```python
from build123d import *

# Parameters (mm, degrees)
SKETCH1_W           = 200
SKETCH1_H           = 120
BOSS_EXTRUDE1_DEPTH = 3
SKETCH2_W           = 5
SKETCH2_H           = 60
CUT_EXTRUDE1_DEPTH  = 117.657618697
SKETCH3_W           = 30
SKETCH3_H           = 3
CUT_EXTRUDE2_DEPTH  = 117.657618697


with BuildPart() as part:
    # Sketch1 → Boss-Extrude1 (new body)
    with BuildSketch(Plane(origin=(0, 0, 0), x_dir=(1, 0, 0), z_dir=(0, 1, 0))):
        Rectangle(SKETCH1_W, SKETCH1_H)
    extrude(amount=BOSS_EXTRUDE1_DEPTH)

    # Sketch2 → Cut-Extrude1 (cut, through all)
    with BuildSketch(Plane(origin=(0, 3, 0), x_dir=(1, 0, 0), z_dir=(0, 1, 0))):
        with Locations((90.5, 0)):
            Rectangle(SKETCH2_W, SKETCH2_H)
    extrude(amount=-CUT_EXTRUDE1_DEPTH, mode=Mode.SUBTRACT)

    # Sketch3 → Cut-Extrude2 (cut, through all)
    with BuildSketch(Plane(origin=(0, 3, 0), x_dir=(1, 0, 0), z_dir=(0, 1, 0))):
        with Locations((70, 41.5)):
            Rectangle(SKETCH3_W, SKETCH3_H)
        with Locations((70, -41.5)):
            Rectangle(SKETCH3_W, SKETCH3_H)
    extrude(amount=-CUT_EXTRUDE2_DEPTH, mode=Mode.SUBTRACT)


solid = part.part
```
Geometry: final body of the model. Coordinates: model frame, mm. Coordinates: 2 decimals unless noted, no trailing zeros. Order: outer loops, then holes, each group sorted by start corner. A loop starts at its lowest first (then second) coordinate and runs counter-clockwise, first axis right, second up. Notation, with made-up numbers: (35.25, 74.25) -> (59.25, 74.25) arc R15 ccw to (59.25, 85.25) -> close; hole circle Ø2 at (81, -36.5). An arc over 180 degrees is marked (long way). Use CSV: the item, a comma, the result in double quotes.
1) Section A-A on x = 58.5. Output: boundary loops of the cut face in (y, z), then the cut area to 3 significant figures.
Findings:
outline,"(0, -60) -> (3, -60) -> (3, -43) -> (0, -43) -> close; (0, -40) -> (3, -40) -> (3, 40) -> (0, 40) -> close; (0, 43) -> (3, 43) -> (3, 60) -> (0, 60) -> close"
area,"342 mm^2"
2) Section C-C on z = 18. Output: boundary loops of the cut face in (x, y).
Findings:
outline,"(-100, 0) -> (88, 0) -> (88, 3) -> (-100, 3) -> close; (93, 0) -> (100, 0) -> (100, 3) -> (93, 3) -> close"
3) Section B-B on y = 1.6. Output: boundary loops of the cut face in (x, z), then the cut area to 3 significant figures.
Findings:
outline,"(-100, -60) -> (100, -60) -> (100, 60) -> (-100, 60) -> close; hole (55, -43) -> (85, -43) -> (85, -40) -> (55, -40) -> close; hole (55, 40) -> (85, 40) -> (85, 43) -> (55, 43) -> close; hole (88, -30) -> (93, -30) -> (93, 30) -> (88, 30) -> close"
area,"23,500 mm^2"
4) Pin query (flat end, axial travel): pin 1 Ø6 at (x, z) = (-33.5, -14) entering from -Y. Return the tip coordinate at first contact, or that it passes through.
Findings:
pin 1,"stops at y = 0"
5) Line query: line 1 (Z direction, x = 63, y = 0.2); line 2 (X direction, y = 1.95, z = -7). Output: solid intervals per line, ascending.
Findings:
line 1,"z = -60 to -43, -40 to 40, 43 to 60"
line 2,"x = -100 to 88, 93 to 100"
